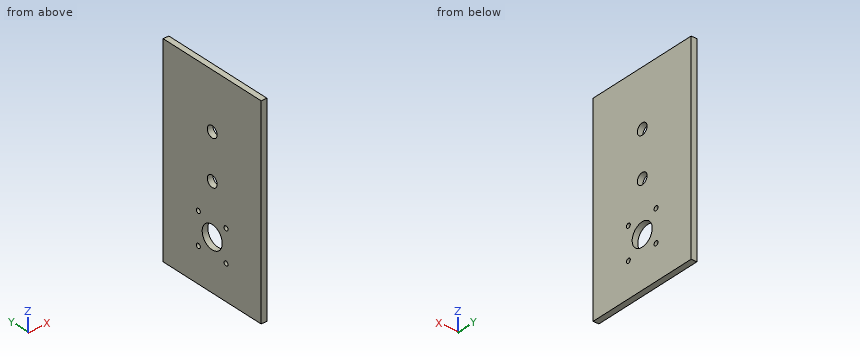
```python
from build123d import *

# Parameters (mm, degrees)
SKETCH2_W           = 228.6
SKETCH2_H           = 127
SKETCH2_R           = 6.35
SKETCH2_R_2         = 13.000000035
SKETCH2_R_3         = 2.5527
BOSS_EXTRUDE2_DEPTH = 6.35


with BuildPart() as part:
    # Sketch2 → Boss-Extrude2 (new body)
    with BuildSketch(Plane(origin=(0, 0, 0), x_dir=(0, 0, -1), z_dir=(1, 0, 0))):
        Rectangle(SKETCH2_W, SKETCH2_H)
        with Locations((-50.8, 0)):
            Circle(SKETCH2_R, mode=Mode.SUBTRACT)
        with Locations((57.15, 0)):
            Circle(SKETCH2_R_2, mode=Mode.SUBTRACT)
        Circle(SKETCH2_R, mode=Mode.SUBTRACT)
        with Locations((75.110512242, 17.960512242)):
            Circle(SKETCH2_R_3, mode=Mode.SUBTRACT)
        with Locations((75.110512242, -17.960512242)):
            Circle(SKETCH2_R_3, mode=Mode.SUBTRACT)
        with Locations((39.189487758, -17.960512242)):
            Circle(SKETCH2_R_3, mode=Mode.SUBTRACT)
        with Locations((39.189487758, 17.960512242)):
            Circle(SKETCH2_R_3, mode=Mode.SUBTRACT)
    extrude(amount=BOSS_EXTRUDE2_DEPTH)


solid = part.part
```
Geometry check sheet. Reference: the model listing, model coordinates, mm. Coordinates: 2 decimals unless noted, no trailing zeros. Loops run counter-clockwise (first coordinate to the right, second up) from the corner with the lowest first, then second, coordinate; pieces in that order, holes last. Notation, with made-up numbers: (35.25, 63.25) - (39.25, 63.25) arc R18 cw to (39.25, 87.25) - close; hole circle Ø9 at (57.25, 29). An arc over 180 degrees is marked (long way). One line per item, written item: value. Start each with the question number.
(1) Cross-section at B-B on x = 1.25. Enter the section's corners in (y, z).
(2) Material ranges on line 1 (Z direction, x = 2, y = -0.5); line 2 (Y direction, x = 2, z = -73.5); line 3 (Y direction, x = 4, z = 50.8), recorded low to high. Write a range as [from, to].
(3) Cross-section at C-C on z = 0. Enter the section's corners in (x, y).
(4) Cross-section at A-A on z = -57.15. Enter the section's corners in (x, y).
Results below:
1. outline: (-63.5, -114.3) - (63.5, -114.3) - (63.5, 114.3) - (-63.5, 114.3) - close; hole circle Ø5.11 at (-17.96, -75.11); hole circle Ø5.11 at (-17.96, -39.19); hole circle Ø26 at (0, -57.15); hole circle Ø12.7 at (0, 0); hole circle Ø12.7 at (0, 50.8); hole circle Ø5.11 at (17.96, -75.11); hole circle Ø5.11 at (17.96, -39.19)
2. line 1: z = [-114.3, -70.14], [-44.16, -6.33], [6.33, 44.47], [57.13, 114.3]
2. line 2: y = [-63.5, -19.94], [-15.98, 15.98], [19.94, 63.5]
2. line 3: y = [-63.5, -6.35], [6.35, 63.5]
3. outline: (0, -63.5) - (6.35, -63.5) - (6.35, -6.35) - (0, -6.35) - close; (0, 6.35) - (6.35, 6.35) - (6.35, 63.5) - (0, 63.5) - close
4. outline: (0, -63.5) - (6.35, -63.5) - (6.35, -13) - (0, -13) - close; (0, 13) - (6.35, 13) - (6.35, 63.5) - (0, 63.5) - close
